Part model, mm, in its own coordinate system. A direction names the side the tool comes from. Coordinates: 2 decimals unless noted, no trailing zeros. Order: outer loops, then holes, each group sorted by start corner. A loop starts at its lowest first (then second) coordinate and runs counter-clockwise, first axis right, second up.
```python
from build123d import *

# Parameters (mm, degrees)
SKETCH1_W             = 70
SKETCH1_H             = 37.5
BOSS_EXTRUDE1_DEPTH   = 85.5
SHELL1_T              = -6
SKETCH4_W             = 58
SKETCH4_H             = 2
BOSS_EXTRUDE2_DEPTH   = 31.5
SKETCH3_W             = 64
SKETCH3_H             = 3
CUT_EXTRUDE2_DEPTH    = 2
BOSS_EXTRUDE3_DEPTH   = 40
SKETCH8_W             = 64
SKETCH8_H             = 79.5
BOSS_EXTRUDE4_DEPTH   = 4.5
SKETCH9_W             = 76.5
SKETCH9_H             = 32.167861311
CUT_EXTRUDE3_DEPTH    = 65
SKETCH14_W            = 85.5
SKETCH14_H            = 35.5
CUT_EXTRUDE4_DEPTH    = 4
M2_TAPPED_HOLE1_D     = 1.6
M2_TAPPED_HOLE1_DEPTH = 4
M2_TAPPED_HOLE1_TIP   = 0.480688495
M2_TAPPED_HOLE2_D     = 1.6
M2_TAPPED_HOLE2_DEPTH = 4
M2_TAPPED_HOLE2_TIP   = 0.480688495
SKETCH17_W            = 12
SKETCH17_H            = 7
CUT_EXTRUDE5_DEPTH    = 10
SKETCH19_W            = 24
SKETCH19_H            = 4
BOSS_EXTRUDE5_DEPTH   = 61
SKETCH20_W            = 5.5
SKETCH20_H            = 9.526840529
BOSS_EXTRUDE7_DEPTH   = 17
SKETCH21_W            = 24
SKETCH21_H            = 4
CUT_EXTRUDE6_DEPTH    = 15.5


with BuildPart() as part:
    # Sketch1 → Boss-Extrude1 (new body)
    with BuildSketch(Plane.XY):
        Rectangle(SKETCH1_W, SKETCH1_H)
    extrude(amount=-BOSS_EXTRUDE1_DEPTH)

    # Shell1
    shell1_openings = [part.faces().sort_by_distance(p)[0] for p in [
        (0, 18.75, -42.75),
    ]]
    offset(amount=SHELL1_T, openings=shell1_openings, kind=Kind.INTERSECTION)

    # Sketch4 → Boss-Extrude2 (add)
    with BuildSketch(Plane(origin=(0, -12.75, 0), x_dir=(1, 0, 0), z_dir=(0, 1, 0))):
        with Locations((0, 78.5)):
            Rectangle(SKETCH4_W, SKETCH4_H)
        with Locations((0, 7)):
            Rectangle(SKETCH4_W, SKETCH4_H)
    extrude(amount=BOSS_EXTRUDE2_DEPTH)

    # Sketch3 → Cut-Extrude2 (cut)
    with BuildSketch(Plane(origin=(0, 18.75, 0), x_dir=(1, 0, 0), z_dir=(0, 1, 0))):
        with Locations((-3, 4.5)):
            Rectangle(SKETCH3_W, SKETCH3_H)
        with Locations((-3, 81)):
            Rectangle(SKETCH3_W, SKETCH3_H)
    extrude(amount=-CUT_EXTRUDE2_DEPTH, mode=Mode.SUBTRACT)

    # Sketch6 → Boss-Extrude3 (add)
    with BuildSketch(Plane(origin=(0, 18.75, 0), x_dir=(1, 0, 0), z_dir=(0, 1, 0))):
        Polygon((29, 79.5), (29, 6), (29, 3), (-35, 3), (-35, 0), (35, 0), (35, 85.5), (-35, 85.5), (-35, 82.5), (29, 82.5), align=None)
    extrude(amount=BOSS_EXTRUDE3_DEPTH)

    # Sketch8 → Boss-Extrude4 (add)
    with BuildSketch(Plane(origin=(0, 58.75, 0), x_dir=(1, 0, 0), z_dir=(0, 1, 0))):
        with Locations((-3, 42.75)):
            Rectangle(SKETCH8_W, SKETCH8_H)
    extrude(amount=-BOSS_EXTRUDE4_DEPTH)

    # Sketch9 → Cut-Extrude3 (cut)
    with BuildSketch(Plane.ZY.offset(35)):
        with Locations((-42.75, -0.972421296)):
            Rectangle(SKETCH9_W, SKETCH9_H)
    extrude(amount=-CUT_EXTRUDE3_DEPTH, mode=Mode.SUBTRACT)

    # Sketch14 → Cut-Extrude4 (cut)
    with BuildSketch(Plane.ZY.offset(35)):
        with Locations((-42.75, -1)):
            Rectangle(SKETCH14_W, SKETCH14_H)
    extrude(amount=-CUT_EXTRUDE4_DEPTH, mode=Mode.SUBTRACT)

    # M2 Tapped Hole1
    with Locations(Plane.ZY.offset(35)):
        with Locations((-2.25, 13.25), (-83.25, -16.5), (-83.25, 13.25), (-2.25, -16.5)):
            Hole(M2_TAPPED_HOLE1_D / 2, depth=M2_TAPPED_HOLE1_DEPTH)
            with Locations((0, 0, -(M2_TAPPED_HOLE1_DEPTH + M2_TAPPED_HOLE1_TIP / 2))):  # 118° drill point
                Cone(0, M2_TAPPED_HOLE1_D / 2, M2_TAPPED_HOLE1_TIP, mode=Mode.SUBTRACT)

    # M2 Tapped Hole2
    with Locations(Plane.ZY.offset(31)):
        with Locations((-2.25, 13.25), (-2.25, -16.5), (-83.25, -16.5), (-83.25, 13.25)):
            Hole(M2_TAPPED_HOLE2_D / 2, depth=M2_TAPPED_HOLE2_DEPTH)
            with Locations((0, 0, -(M2_TAPPED_HOLE2_DEPTH + M2_TAPPED_HOLE2_TIP / 2))):  # 118° drill point
                Cone(0, M2_TAPPED_HOLE2_D / 2, M2_TAPPED_HOLE2_TIP, mode=Mode.SUBTRACT)

    # Sketch17 → Cut-Extrude5 (cut)
    with BuildSketch(Plane(origin=(35, 0, 0), x_dir=(0, 0, -1), z_dir=(1, 0, 0))):
        with Locations((42.75, -10.993248875)):
            Rectangle(SKETCH17_W, SKETCH17_H)
    extrude(amount=-CUT_EXTRUDE5_DEPTH, mode=Mode.SUBTRACT)

    # Sketch19 → Boss-Extrude5 (add)
    with BuildSketch(Plane.ZY.offset(31)):
        with Locations((-69, 0.411509359)):
            Rectangle(SKETCH19_W, SKETCH19_H)
    extrude(amount=-BOSS_EXTRUDE5_DEPTH)

    # Sketch20 → Boss-Extrude7 (add)
    with BuildSketch(Plane.XY.offset(-81)):
        with Locations((16.25, 7.174929624)):
            Rectangle(SKETCH20_W, SKETCH20_H)
        with Locations((-12.75, 7.174929624)):
            Rectangle(SKETCH20_W, SKETCH20_H)
    extrude(amount=BOSS_EXTRUDE7_DEPTH)

    # Sketch21 → Cut-Extrude6 (cut)
    with BuildSketch(Plane.ZY.offset(31)):
        with Locations((-69, 0.411509359)):
            Rectangle(SKETCH21_W, SKETCH21_H)
    extrude(amount=-CUT_EXTRUDE6_DEPTH, mode=Mode.SUBTRACT)


solid = part.part
```
(1) Slice it at B-B, the plane x = 10.5. Give the cut face in (y, z), then the cut area to 3 significant figures.
(2) Slice it at A-A, the plane z = -35. Give the cut face in (x, y).
(3) Slice it at C-C, the plane y = 8. Give the cut face in (x, z).
(4) Slice it at D-D, the plane z = -72. Give the cut face in (x, y), then the cut area to 3 significant figures.
(5) Tool access for faces 5 (the face through (-3, 35, -82.5)), 6 (the face through (-33, 16.75, -2)), 7 (the face through (-29, 17, -42)), 8 (the face through (0, 19, 0)): list every direction of +Z, -Z, +X, -X, +Y, -Y with a clear straight run to the whole face (end or side of a thin tool).
(6) Drop flat-ended pins along their axis: pin 1 (1.2 mm diameter, centred on x = -32.5, z = -25.5, fed in from -Y); pin 2 (4 mm diameter, centred on y = 48, z = -40.5, fed in from -X). Give the stop position or say it passes through.
(7) Pull direction X, two halves, no side cores. Call faces 1 (the face through (-13, 7, -64)), 2 (the face through (0, 17, -77.5)), 3 (the face through (13.5, 7, -73)), 4 (the face through (35, 19, -42)): +X half, -X half, draft (parallel to the pull), parting line (faces both ways), or undercut.
(8) Probe line 1 (Z direction, x = -28.4, y = 13.25); line 2 (Y direction, x = -28.1, z = -83.25); line 3 (Y direction, x = -11, z = -75). List the from-to ranges inside material, lowest first.
Here are the results:
1. outline: (-18.75, -85.5) - (58.75, -85.5) - (58.75, 0) - (-18.75, 0) - close; hole (-17.06, -81) - (-1.59, -81) - (-1.59, -57) - (2.41, -57) - (2.41, -81) - (15.11, -81) - (15.11, -77.5) - (18.75, -77.5) - (18.75, -79.5) - (16.75, -79.5) - (16.75, -82.5) - (54.25, -82.5) - (54.25, -3) - (16.75, -3) - (16.75, -6) - (18.75, -6) - (18.75, -8) - (15.11, -8) - (15.11, -4.5) - (-17.06, -4.5) - close
1. area: 1,170 mm2
2. outline: (-35, 16.75) - (-31, 16.75) - (-31, 15.11) - (-29, 15.11) - (-29, 18.75) - (-35, 18.75) - close; (-35, 54.25) - (29, 54.25) - (29, 15.11) - (30, 15.11) - (30, -17.06) - (-31, -17.06) - (-31, -18.75) - (35, -18.75) - (35, 58.75) - (-35, 58.75) - close
3. outline: (-31, -85.5) - (35, -85.5) - (35, 0) - (-31, 0) - (-31, -4.5) - (30, -4.5) - (30, -81) - (19, -81) - (19, -64) - (13.5, -64) - (13.5, -81) - (-10, -81) - (-10, -64) - (-15.5, -64) - (-15.5, -81) - (-31, -81) - close
4. outline: (-35, 16.75) - (-31, 16.75) - (-31, 15.11) - (-29, 15.11) - (-29, 18.75) - (-35, 18.75) - close; (-35, 54.25) - (29, 54.25) - (29, 15.11) - (30, 15.11) - (30, 2.41) - (19, 2.41) - (19, 11.94) - (13.5, 11.94) - (13.5, 2.41) - (-10, 2.41) - (-10, 11.94) - (-15.5, 11.94) - (-15.5, -1.59) - (30, -1.59) - (30, -17.06) - (-31, -17.06) - (-31, -18.75) - (35, -18.75) - (35, 58.75) - (-35, 58.75) - close
4. area: 1,120 mm2
5. face 5: -X
5. face 6: +Z, -Z, -X, -Y
5. face 7: none
5. face 8: +Z, +X, -X, +Y, -Y
6. pin 1: stops at y = 16.75
6. pin 2: stops at x = 29
7. face 1: draft
7. face 2: undercut
7. face 3: undercut
7. face 4: +X half
8. line 1: z = -85.5 to -84.05, -82.45 to -81, -4.5 to -3.05, -1.45 to 0
8. line 2: y = -18.75 to -17.3, -15.7 to 12.45, 14.05 to 58.75
8. line 3: y = -18.75 to -17.06, -1.59 to 11.94, 54.25 to 58.75
